from build123d import *

# Parameters (mm, degrees)
SKETCH1_W           = 25.4
SKETCH1_H           = 76.2
BOSS_EXTRUDE1_DEPTH = 88.9
SHELL1_T            = -3.175
SKETCH2_W           = 25.4
SKETCH2_H           = 25.4
CUT_EXTRUDE1_DEPTH  = 100.9999
SKETCH3_R           = 2.38125
CUT_EXTRUDE2_DEPTH  = 118.774954893


with BuildPart() as part:
    # Sketch1 → Boss-Extrude1 (new, symmetric)
    with BuildSketch(Plane.XY):
        Rectangle(SKETCH1_W, SKETCH1_H)
    extrude(amount=BOSS_EXTRUDE1_DEPTH, both=True)

    # Shell1
    shell1_openings = [part.faces().sort_by_distance(p)[0] for p in [
        (0, 0, 88.9),
        (0, 0, -88.9),
    ]]
    offset(amount=SHELL1_T, openings=shell1_openings, kind=Kind.INTERSECTION)

    # Sketch2 → Cut-Extrude1 (cut, through all)
    with BuildSketch(Plane.ZY.offset(12.7)):
        with Locations((-76.2, 25.4)):
            Rectangle(SKETCH2_W, SKETCH2_H)
    extrude(amount=-CUT_EXTRUDE1_DEPTH, mode=Mode.SUBTRACT)

    # Sketch3 → Cut-Extrude2 (cut, through all)
    with BuildSketch(Plane(origin=(0, 38.1, 0), x_dir=(1, 0, 0), z_dir=(0, 1, 0))):
        with Locations((0, -88.9)):
            Circle(SKETCH3_R)
        with Locations(Location((0, -75.995900078, 0), (0, 0, 270))):
            Circle(SKETCH3_R)
        with Locations(Location((0, -63.397337518, 0), (0, 0, 270))):
            Circle(SKETCH3_R)
        with Locations(Location((0, -50.731481722, 0), (0, 0, 270))):
            Circle(SKETCH3_R)
        with Locations(Location((0, -38.048590908, 0), (0, 0, 270))):
            Circle(SKETCH3_R)
        with Locations(Location((0, 63.5, 0), (0, 0, 270))):
            Circle(SKETCH3_R)
        with Locations(Location((0, 12.648590908, 0), (0, 0, 270))):
            Circle(SKETCH3_R)
        with Locations(Location((0, 25.331481722, 0), (0, 0, 270))):
            Circle(SKETCH3_R)
        with Locations(Location((0, 37.997337518, 0), (0, 0, 270))):
            Circle(SKETCH3_R)
        with Locations(Location((0, 50.595900078, 0), (0, 0, 270))):
            Circle(SKETCH3_R)
    extrude(amount=-CUT_EXTRUDE2_DEPTH, mode=Mode.SUBTRACT)


solid = part.part
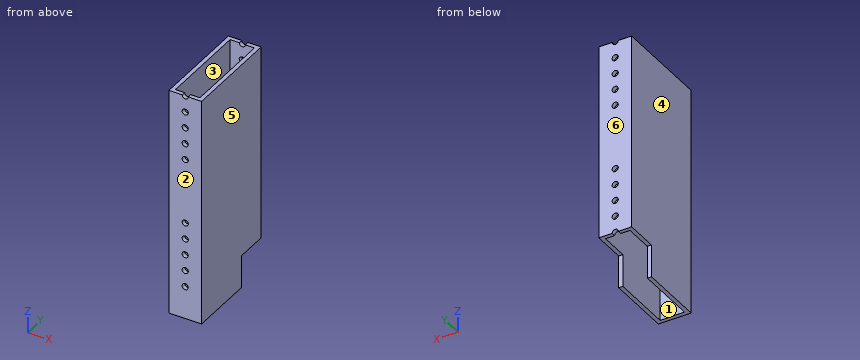
For this review, take the finished solid that the model builds, in its own axes (mm). Face numbers are marked on the shaded views. A direction names the side the tool comes from. Give positions to 0.01 mm unless a question says otherwise; leave off trailing zeros. Order: outer loops, then holes, each group sorted by start corner. A loop starts at its lowest first (then second) coordinate and runs counter-clockwise, first axis right, second up. Notation, with made-up numbers: M -11.5,13 L 37.5,13 A34 cw 37.5,43 Z; hole C -8,24 d6. An arc over 180 degrees is marked long. Answer in a Markdown table with one row per item. Add a question column.
(1) Consider section A-A on y = -2.5. State the section outline as (x, z) points (3 decimals), and give its area (3 significant figures).
(2) Consider section C-C on z = -69. State the section outline as (x, y) points (3 decimals).
(3) For pin 1 (11.5 mm diameter, centred on x = -6.5, y = 26, fed in from -Z); pin 2 (1.6 mm diameter, centred on x = 11, z = -82.5, fed in from +Y), all flat-tipped, find the tip position at first contact; note any pin that passes through.
(4) For the marked faces 1 and 2, list the 3-axis set-ups (+Z, -Z, +X, -X, +Y, -Y) from which the entire face can be reached by the end or side of a thin tool; tool diameter is ignored.
(5) Wall thickness on probe 1 along X at (y, z) = (10.5, 77) (3 decimals); probe 2 along Y at (x, z) = (6, -49) (3 decimals); probe 3 along Y at (x, z) = (-7.5, -78.5) (3 decimals): over which ranges is each line inside the solid? List them lowest first. Write a range as [from, to].
(6) Consider section B-B on z = 7. State the section outline as (x, y) points (3 decimals), and give its area (3 significant figures).
(7) Consider section D-D on x = 0. Give the number of separate pieces and of enclosed holes in the cut face, and give its area (3 significant figures).
(8) Mouldability with a two-part tool opening along X and no side actions: class the marked faces 3, 4, 5 and 6 as +X half, -X half, draft (parallel to the pull), parting line (faces both ways), or undercut.
Evaluation:
| question | item | result |
|---|---|---|
| 1 | outline | M -12.7,-88.9 L -9.525,-88.9 L -9.525,88.9 L -12.7,88.9 Z; M 9.525,-88.9 L 12.7,-88.9 L 12.7,88.9 L 9.525,88.9 Z |
| 1 | area | 1,130 mm^2 |
| 2 | outline | M -12.7,-38.1 L 12.7,-38.1 L 12.7,12.7 L 9.525,12.7 L 9.525,-34.925 L -9.525,-34.925 L -9.525,12.7 L -12.7,12.7 Z |
| 3 | pin 1 | stops at z = -63.5 |
| 3 | pin 2 | stops at y = 12.7 |
| 4 | face 1 | +Z, -Z |
| 4 | face 2 | +Z, -Z, +X, -X, -Y |
| 5 | probe 1 | x = [-12.7, -9.525], [9.525, 12.7] |
| 5 | probe 2 | y = [-38.1, -34.925], [34.925, 38.1] |
| 5 | probe 3 | y = [-38.1, -34.925] |
| 6 | outline | M -12.7,-38.1 L 12.7,-38.1 L 12.7,38.1 L -12.7,38.1 Z; hole M -9.525,-34.925 L 9.525,-34.925 L 9.525,34.925 L -9.525,34.925 Z |
| 6 | area | 605 mm^2 |
| 7 | separate pieces | 19 |
| 7 | enclosed holes | 0 |
| 7 | area | 769 mm^2 |
| 8 | face 3 | undercut |
| 8 | face 4 | -X half |
| 8 | face 5 | +X half |
| 8 | face 6 | draft |
